The model under review builds one solid part; all positions refer to its coordinate system, in mm. Coordinates: 2 decimals unless noted, no trailing zeros. Loops run counter-clockwise (first coordinate to the right, second up) from the corner with the lowest first, then second, coordinate; pieces in that order, holes last. Notation, with made-up numbers: M -24.75,6.5 L -5.75,6.5 A13 ccw -5.75,15.5 Z; hole C 27.25,6 d5. An arc over 180 degrees is marked long. Return JSON: item names as keys, results as strings.
```python
from build123d import *

# Parameters (mm, degrees)
F1_DEPTH = 25.4


# Not quite as in the source:
# - the program builds the solid bodies; features that only make, move or delete a surface that nothing else refers to are left out


with BuildPart() as f1:
    # F0 (on Top) → F1 (new body)
    with BuildSketch(Plane.XY):
        with BuildLine():
            ThreePointArc((19.282356954, 0), (17.3548102292, 8.4035618406), (11.957541655, 15.127011842))
            ThreePointArc((11.957541655, 15.127011842), (-18.7957142624, 4.3046968609), (4.1820366195, -18.823385971))
            ThreePointArc((4.1820366195, -18.823385971), (15.0407581689, -12.0658560991), (19.282356954, 0))
        make_face()
        with BuildLine():
            Line((11.957541655, 15.127011842), (17.5544340163, 22.2074184567))
            Line((17.5544340163, 22.2074184567), (35.1088680327, 44.4148369133))
            Line((35.1088680327, 44.4148369133), (-50.3368154168, 57.9507872462))
            Line((-50.3368154168, 57.9507872462), (-64.9315572131, -34.1785170794))
            Line((-64.9315572131, -34.1785170794), (4.1820366195, -18.823385971))
            ThreePointArc((4.1820366195, -18.823385971), (-18.7957142624, 4.3046968609), (11.957541655, 15.127011842))
        make_face()
    extrude(amount=F1_DEPTH)


solid = f1.part
```
1. Add section B-B on z = 19.25. Give the boundary of the cut face in (x, y).
Check values:
{"outline": "M -64.93,-34.18 L 4.18,-18.82 A19.28 ccw 11.96,15.13 L 35.11,44.41 L -50.34,57.95 Z"}
2. Add section A-A on x = 14. Give the boundary of the cut face in (y, z), plus the area to 3 significant figures.
Check values:
{"outline": "M -13.26,0 L 13.26,0 L 13.26,25.4 L -13.26,25.4 Z; M 17.71,0 L 47.76,0 L 47.76,25.4 L 17.71,25.4 Z", "area": "1,440 mm²"}
3. To check wall thickness, follow line 1 (Y direction, x = 17, z = 1.75); line 2 (Y direction, x = -34, z = 10); line 3 (Y direction, x = -6, z = 5.25). State the ranges of each line that lie inside material, in increasing order.
Check values:
{"line 1": "-9.1 to 9.1, 21.51 to 47.28", "line 2": "-27.31 to 55.36", "line 3": "-21.09 to 50.93"}
4. Add section D-D on x = -8. Give the boundary of the cut face in (y, z).
Check values:
{"outline": "M -21.53,0 L 51.24,0 L 51.24,25.4 L -21.53,25.4 Z"}
5. Add section C-C on y = -4. Give the boundary of the cut face in (x, z), plus the area to 3 significant figures.
Check values:
{"outline": "M -60.15,0 L 18.86,0 L 18.86,25.4 L -60.15,25.4 Z", "area": "2,010 mm²"}
6. Insertion check: pin 1 Ø10 at (x, z) = (10, 12) entering from -Y; pin 2 Ø5 at (x, z) = (-48.5, 13) entering from +Y; pin 3 Ø1 at (x, z) = (-8.5, 17) entering from -Y; pin 4 Ø1.5 at (x, z) = (-40, 10.5) entering from +Y. Each pin has a flat end and moves straight along its axis. Give the tip position at first contact, or say it passes through.
Check values:
{"pin 1": "y = -18.62", "pin 2": "y = 57.95", "pin 3": "y = -21.75", "pin 4": "y = 56.43"}
